Geometry check sheet. Reference: the model listing, model coordinates, mm. Round coordinates to 2 decimals unless told otherwise and drop trailing zeros. Loops run counter-clockwise (first coordinate to the right, second up) from the corner with the lowest first, then second, coordinate; pieces in that order, holes last. Notation, with made-up numbers: (19, 48) - (62, 48) arc R30 ccw to (62, 74) - close; hole circle Ø11 at (68.25, 84.25). An arc over 180 degrees is marked (long way). Write item = value, one per line.
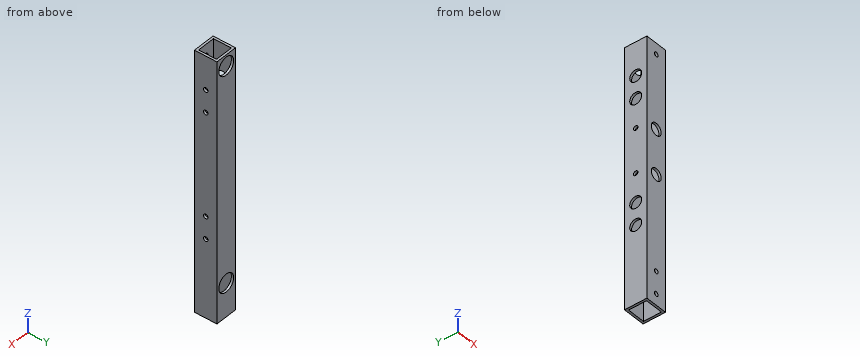
```python
from build123d import *

# Parameters (mm, degrees)
SKETCH_1_W           = 15
SKETCH_1_H           = 15
SKETCH_1_W_2         = 12
SKETCH_1_H_2         = 12
EXTRUDE_2_DEPTH      = 174
CUT_EXTRUDE_1_DEPTH  = 10
SKETCH_3_R           = 1.5
CUT_EXTRUDE_2_DEPTH  = 10
SKETCH_6_R           = 4
CUT_EXTRUDE_4_DEPTH  = 10
SKETCH_7_R           = 1.5
CUT_EXTRUDE_5_DEPTH  = 10
SKETCH_8_R           = 4
CUT_EXTRUDE_6_DEPTH  = 10
SKETCH_10_R          = 1.5
CUT_EXTRUDE_9_DEPTH  = 10
SKETCH_12_R          = 4
CUT_EXTRUDE_10_DEPTH = 10
SKETCH_13_R          = 1.5
CUT_EXTRUDE_11_DEPTH = 10
SKETCH_14_R          = 4
CUT_EXTRUDE_12_DEPTH = 10
SKETCH_15_R          = 1.5
CUT_EXTRUDE_13_DEPTH = 10
SKETCH_16_R          = 6
CUT_EXTRUDE_14_DEPTH = 10
SKETCH_17_R          = 1.5
CUT_EXTRUDE_15_DEPTH = 10
SKETCH_18_R          = 6
CUT_EXTRUDE_16_DEPTH = 10
SKETCH_19_R          = 4
CUT_EXTRUDE_17_DEPTH = 10
SKETCH_20_R          = 1.5
CUT_EXTRUDE_18_DEPTH = 10
SKETCH_21_R          = 1.5
CUT_EXTRUDE_19_DEPTH = 10
SKETCH_22_R          = 4
CUT_EXTRUDE_20_DEPTH = 10


with BuildPart() as part:
    # ｽｹｯﾁ1 → ﾎﾞｽ - 押し出し2 (new body)
    with BuildSketch(Plane.XY):
        with Locations((0.489915859, 0.232626086)):
            Rectangle(SKETCH_1_W, SKETCH_1_H)
        with Locations((0.489915859, 0.232626086)):
            Rectangle(SKETCH_1_W_2, SKETCH_1_H_2, mode=Mode.SUBTRACT)
    extrude(amount=EXTRUDE_2_DEPTH)

    # ｽｹｯﾁ2 → ｶｯﾄ - 押し出し1 (cut)
    with BuildSketch(Plane(origin=(0, -7.267373914, 0), x_dir=(-1, 0, 0), z_dir=(0, -1, 0))):
        with BuildLine():
            ThreePointArc((1.010084141, -7.5), (0.570744313, -6.439339828), (-0.489915859, -6))
            Line((-0.489915859, -6), (-0.489915859, -7.5))
            Line((-0.489915859, -7.5), (1.010084141, -7.5))
        make_face()
        with BuildLine():
            Line((-0.489915859, -7.5), (-0.489915859, -6))
            ThreePointArc((-0.489915859, -6), (-1.550576031, -8.560660172), (1.010084141, -7.5))
            Line((1.010084141, -7.5), (-0.489915859, -7.5))
        make_face()
    extrude(amount=-CUT_EXTRUDE_1_DEPTH, mode=Mode.SUBTRACT)

    # ｽｹｯﾁ3 → ｶｯﾄ - 押し出し2 (cut)
    with BuildSketch(Plane(origin=(7.989915859, 0, 0), x_dir=(0, 0, -1), z_dir=(1, 0, 0))):
        with Locations((-52.5, 0.232626086)):
            Circle(SKETCH_3_R)
    extrude(amount=-CUT_EXTRUDE_2_DEPTH, mode=Mode.SUBTRACT)

    # ｽｹｯﾁ6 → ｶｯﾄ - 押し出し4 (cut)
    with BuildSketch(Plane.ZY.offset(7.010084141)):
        with Locations((52.5, 0.232626086)):
            Circle(SKETCH_6_R)
    extrude(amount=-CUT_EXTRUDE_4_DEPTH, mode=Mode.SUBTRACT)

    # ｽｹｯﾁ7 → ｶｯﾄ - 押し出し5 (cut)
    with BuildSketch(Plane(origin=(7.989915859, 0, 0), x_dir=(0, 0, -1), z_dir=(1, 0, 0))):
        with Locations((-151.5, 0.232626086)):
            Circle(SKETCH_7_R)
    extrude(amount=-CUT_EXTRUDE_5_DEPTH, mode=Mode.SUBTRACT)

    # ｽｹｯﾁ8 → ｶｯﾄ - 押し出し6 (cut)
    with BuildSketch(Plane.ZY.offset(7.010084141)):
        with Locations((151.5, 0.232626086)):
            Circle(SKETCH_8_R)
    extrude(amount=-CUT_EXTRUDE_6_DEPTH, mode=Mode.SUBTRACT)

    # ｽｹｯﾁ10 → ｶｯﾄ - 押し出し9 (cut)
    with BuildSketch(Plane.ZY.offset(7.010084141)):
        with Locations((86.8, 0.232626086)):
            Circle(SKETCH_10_R)
    extrude(amount=-CUT_EXTRUDE_9_DEPTH, mode=Mode.SUBTRACT)

    # ｽｹｯﾁ12 → ｶｯﾄ - 押し出し10 (cut)
    with BuildSketch(Plane.XZ.offset(7.267373914)):
        with Locations((0.489915859, 86.8)):
            Circle(SKETCH_12_R)
    extrude(amount=-CUT_EXTRUDE_10_DEPTH, mode=Mode.SUBTRACT)

    # ｽｹｯﾁ13 → ｶｯﾄ - 押し出し11 (cut)
    with BuildSketch(Plane.ZY.offset(7.010084141)):
        with Locations((116.8, 0.232626086)):
            Circle(SKETCH_13_R)
    extrude(amount=-CUT_EXTRUDE_11_DEPTH, mode=Mode.SUBTRACT)

    # ｽｹｯﾁ14 → ｶｯﾄ - 押し出し12 (cut)
    with BuildSketch(Plane.XZ.offset(7.267373914)):
        with Locations((0.489915859, 116.8)):
            Circle(SKETCH_14_R)
    extrude(amount=-CUT_EXTRUDE_12_DEPTH, mode=Mode.SUBTRACT)

    # ｽｹｯﾁ15 → ｶｯﾄ - 押し出し13 (cut)
    with BuildSketch(Plane.XZ.offset(7.267373914)):
        with Locations((0.489915859, 22.5)):
            Circle(SKETCH_15_R)
    extrude(amount=-CUT_EXTRUDE_13_DEPTH, mode=Mode.SUBTRACT)

    # ｽｹｯﾁ16 → ｶｯﾄ - 押し出し14 (cut)
    with BuildSketch(Plane(origin=(0, 7.732626086, 0), x_dir=(1, 0, 0), z_dir=(0, 1, 0))):
        with Locations((0.489915859, -22.5)):
            Circle(SKETCH_16_R)
    extrude(amount=-CUT_EXTRUDE_14_DEPTH, mode=Mode.SUBTRACT)

    # ｽｹｯﾁ17 → ｶｯﾄ - 押し出し15 (cut)
    with BuildSketch(Plane.XZ.offset(7.267373914)):
        with Locations((0.489915859, 166.5)):
            Circle(SKETCH_17_R)
    extrude(amount=-CUT_EXTRUDE_15_DEPTH, mode=Mode.SUBTRACT)

    # ｽｹｯﾁ18 → ｶｯﾄ - 押し出し16 (cut)
    with BuildSketch(Plane(origin=(0, 7.732626086, 0), x_dir=(1, 0, 0), z_dir=(0, 1, 0))):
        with Locations((0.489915859, -166.5)):
            Circle(SKETCH_18_R)
    extrude(amount=-CUT_EXTRUDE_16_DEPTH, mode=Mode.SUBTRACT)

    # ｽｹｯﾁ19 → ｶｯﾄ - 押し出し17 (cut)
    with BuildSketch(Plane.ZY.offset(7.010084141)):
        with Locations((67.5, 0.232626086)):
            Circle(SKETCH_19_R)
    extrude(amount=-CUT_EXTRUDE_17_DEPTH, mode=Mode.SUBTRACT)

    # ｽｹｯﾁ20 → ｶｯﾄ - 押し出し18 (cut)
    with BuildSketch(Plane(origin=(7.989915859, 0, 0), x_dir=(0, 0, -1), z_dir=(1, 0, 0))):
        with Locations((-67.5, 0.232626086)):
            Circle(SKETCH_20_R)
    extrude(amount=-CUT_EXTRUDE_18_DEPTH, mode=Mode.SUBTRACT)

    # ｽｹｯﾁ21 → ｶｯﾄ - 押し出し19 (cut)
    with BuildSketch(Plane(origin=(7.989915859, 0, 0), x_dir=(0, 0, -1), z_dir=(1, 0, 0))):
        with Locations((-136.5, 0.232626086)):
            Circle(SKETCH_21_R)
    extrude(amount=-CUT_EXTRUDE_19_DEPTH, mode=Mode.SUBTRACT)

    # ｽｹｯﾁ22 → ｶｯﾄ - 押し出し20 (cut)
    with BuildSketch(Plane.ZY.offset(7.010084141)):
        with Locations((136.5, 0.232626086)):
            Circle(SKETCH_22_R)
    extrude(amount=-CUT_EXTRUDE_20_DEPTH, mode=Mode.SUBTRACT)


solid = part.part
```
(1) Scan lines: L1, parallel to Y at x = 7.25, z = 151.5; L2, parallel to X at y = -6.6, z = 7.5; L3, parallel to Y at x = -2.25, z = 80. Record each from-to range of solid material in increasing order. Write a range as [from, to].
Answers follow:
L1 = [-7.27, -1.27], [1.73, 7.73]
L2 = [-7.01, -1.01], [1.99, 7.99]
L3 = [-7.27, -5.77], [6.23, 7.73]
(2) Section check A-A (z = 38). Enter the section's corners in (x, y), then the cut area to 3 significant figures.
Answers follow:
outline = (-7.01, -7.27) - (7.99, -7.27) - (7.99, 7.73) - (-7.01, 7.73) - close; hole (-5.51, -5.77) - (6.49, -5.77) - (6.49, 6.23) - (-5.51, 6.23) - close
area = 81.0 mm²
(3) Section check B-B (z = 151.5). Enter the section's corners in (x, y), then the cut area to 3 significant figures.
Answers follow:
outline = (-7.01, -7.27) - (7.99, -7.27) - (7.99, -1.27) - (6.49, -1.27) - (6.49, -5.77) - (-5.51, -5.77) - (-5.51, -3.77) - (-7.01, -3.77) - close; (-7.01, 4.23) - (-5.51, 4.23) - (-5.51, 6.23) - (6.49, 6.23) - (6.49, 1.73) - (7.99, 1.73) - (7.99, 7.73) - (-7.01, 7.73) - close
area = 64.5 mm²
(4) Gauge pin test, flat end, axial feed: pin 1 (1.8 mm diameter, centred on y = 0.23, z = 86.8, fed in from -X). Record the tip position at first contact, or that the pin passes through.
Answers follow:
pin_1 = 6.49
